Geometry check sheet. Reference: the model listing, model coordinates, mm. Coordinates: 2 decimals unless noted, no trailing zeros. Write each loop counter-clockwise with the first axis right and the second up, starting at its lowest first coordinate (ties: lowest second). Pieces come first, ordered by that corner, then holes.
from build123d import *

# Parameters (mm, degrees)
BOSS_EXTRUDE1_OUTLINE_W   = 142
BOSS_EXTRUDE1_OUTLINE_H   = 46
BOSS_EXTRUDE1_OUTLINE_R   = 1.6
BOSS_EXTRUDE1_OUTLINE_R_2 = 1.5
BOSS_EXTRUDE1_DEPTH       = 3
FILLET4_R                 = 6
SKETCH3_R                 = 2
SKETCH3_R_2               = 1.5
BOSS_EXTRUDE2_DEPTH       = 3
SKETCH3_7_R               = 1.5
SKETCH3_7_R_2             = 2
CUT_EXTRUDE1_DEPTH        = 3
FILLET5_R                 = 10
SKETCH2_3_R               = 1.5
CUT_EXTRUDE2_DEPTH        = 10


# Read off the part's stored shape, not the designer's step: Boss-Extrude1
with BuildPart() as part:
    # Boss-Extrude1 outline → Boss-Extrude1 (new body)
    with BuildSketch(Plane.XY):
        with Locations((15, 0)):
            Rectangle(BOSS_EXTRUDE1_OUTLINE_W, BOSS_EXTRUDE1_OUTLINE_H)
        with Locations((-45, -14)):
            Circle(BOSS_EXTRUDE1_OUTLINE_R, mode=Mode.SUBTRACT)
        with Locations((15, -14)):
            Circle(BOSS_EXTRUDE1_OUTLINE_R, mode=Mode.SUBTRACT)
        with Locations((42, -11)):
            Circle(BOSS_EXTRUDE1_OUTLINE_R_2, mode=Mode.SUBTRACT)
        with Locations((-45, 14)):
            Circle(BOSS_EXTRUDE1_OUTLINE_R, mode=Mode.SUBTRACT)
        with Locations((42, 11)):
            Circle(BOSS_EXTRUDE1_OUTLINE_R_2, mode=Mode.SUBTRACT)
        with Locations((15, 14)):
            Circle(BOSS_EXTRUDE1_OUTLINE_R, mode=Mode.SUBTRACT)
    extrude(amount=BOSS_EXTRUDE1_DEPTH)

    # Fillet4
    fillet4_edges = [part.edges().sort_by_distance(p)[0] for p in [
        (-56, -23, 1.5),
        (-56, 23, 1.5),
    ]]
    fillet(fillet4_edges, radius=FILLET4_R)

    # Sketch3 → Boss-Extrude2 (add)
    with BuildSketch(Plane.XY.offset(3)):
        Polygon((131, -23), (131, 23), (86, 23), (86, -19), (86, -23), align=None)
        with Locations((93, -19)):
            Circle(SKETCH3_R, mode=Mode.SUBTRACT)
        with Locations((116, -18.25)):
            Circle(SKETCH3_R_2, mode=Mode.SUBTRACT)
        with BuildLine():
            ThreePointArc((110, 0), (120.242640687, 4.242640687), (116, -6))
            ThreePointArc((116, -6), (111.757359313, -4.242640687), (110, 0))
        make_face(mode=Mode.SUBTRACT)
        with Locations((105, 19)):
            Circle(SKETCH3_R, mode=Mode.SUBTRACT)
        with Locations((116, 18.25)):
            Circle(SKETCH3_R_2, mode=Mode.SUBTRACT)
        with Locations((93, 19)):
            Circle(SKETCH3_R, mode=Mode.SUBTRACT)
    extrude(amount=-BOSS_EXTRUDE2_DEPTH)

    # Sketch3<7> → Cut-Extrude1 (cut)
    with BuildSketch(Plane.XY.offset(3)):
        with Locations((51, 19)):
            Circle(SKETCH3_7_R)
        with Locations((-49, 19)):
            Circle(SKETCH3_7_R)
        with Locations((69, -19)):
            Circle(SKETCH3_7_R_2)
        with Locations((81, -19)):
            Circle(SKETCH3_7_R_2)
        with Locations((69, 19)):
            Circle(SKETCH3_7_R_2)
        with Locations((81, 19)):
            Circle(SKETCH3_7_R_2)
        with Locations((-49, -19)):
            Circle(SKETCH3_7_R)
        with Locations((51, -19)):
            Circle(SKETCH3_7_R)
    extrude(amount=-CUT_EXTRUDE1_DEPTH, mode=Mode.SUBTRACT)

    # Fillet5
    fillet5_edges = [part.edges().sort_by_distance(p)[0] for p in [
        (131, 23, 1.5),
        (131, -23, 1.5),
    ]]
    fillet(fillet5_edges, radius=FILLET5_R)

    # Sketch2<3> → Cut-Extrude2 (cut)
    with BuildSketch(Plane.XY):
        with Locations((102, 11)):
            Circle(SKETCH2_3_R)
        with Locations(Location((102, -11, 0), (0, 0, 180))):
            Circle(SKETCH2_3_R)
    extrude(amount=CUT_EXTRUDE2_DEPTH, mode=Mode.SUBTRACT)


solid = part.part
1. Gauge pin test, flat ends, axial feed: pin 1 Ø5 at (x, y) = (42, -11) entering from +Z; pin 2 Ø1.9 at (x, y) = (-45, 14) entering from +Z. Record the tip position at first contact, or that the pin passes through.
Computed values:
pin 1: stops at z = 3
pin 2: passes through
2. Sectioned sample at A-A, the plane z = 1.45. Give the number of separate pieces and of enclosed holes in the cut face, and give its area (3 significant figures).
Computed values:
separate pieces: 1
enclosed holes: 22
area: 8,240 mm2
3. Thickness scan on line 1 along Y through (x, z) = (51, 0.7); line 2 along Y through (x, z) = (93, 2.85); line 3 along X through (y, z) = (3, 2.9). Record the ranges inside material, lowest first.
Computed values:
line 1: y = -23 to -20.5, -17.5 to 17.5, 20.5 to 23
line 2: y = -23 to -21, -17 to 17, 21 to 23
line 3: x = -56 to 110.8, 121.2 to 131
4. Sectioned sample at B-B, the plane x = 15. Record the boundary of the cut face in (y, z), and give its area (3 significant figures).
Computed values:
outline: (-23, 0) - (-15.6, 0) - (-15.6, 3) - (-23, 3) - close; (-12.4, 0) - (12.4, 0) - (12.4, 3) - (-12.4, 3) - close; (15.6, 0) - (23, 0) - (23, 3) - (15.6, 3) - close
area: 119 mm2
5. Sectioned sample at C-C, the plane y = 4. Record the boundary of the cut face in (x, z).
Computed values:
outline: (-56, 0) - (111.53, 0) - (111.53, 3) - (-56, 3) - close; (120.47, 0) - (131, 0) - (131, 3) - (120.47, 3) - close
6. Draft check along Y on faces 1 (the cylindrical face through (101.194, -12.265, 1.479)), 2 (the cylindrical face through (-54.289, -21.196, 1.521)), 3 (the cylindrical face through (94.908, -18.399, 1.521)), 4 (the flat face through (131, 0, 2)). Enter one of: released by +Y, released by -Y, zero draft, split by the parting line, or undercut.
Computed values:
face 1: undercut
face 2: released by -Y
face 3: undercut
face 4: zero draft
